from build123d import *

# Parameters (mm, degrees)
SKETCH1_W           = 152.25
SKETCH1_H           = 51
SKETCH1_R           = 1.75
SKETCH1_R_2         = 2
BOSS_EXTRUDE1_DEPTH = 1.5


with BuildPart() as part:
    # Sketch1 → Boss-Extrude1 (new body)
    with BuildSketch(Plane(origin=(0, 0, 0), x_dir=(1, 0, 0), z_dir=(0, 1, 0))):
        Rectangle(SKETCH1_W, SKETCH1_H)
        with Locations(Location((-63.125, 12.5, 0), (0, 0, 270))):
            Circle(SKETCH1_R, mode=Mode.SUBTRACT)
        with Locations(Location((-63.125, -13, 0), (0, 0, 270))):
            Circle(SKETCH1_R, mode=Mode.SUBTRACT)
        with Locations(Location((-28.125, 12.5, 0), (0, 0, 270))):
            Circle(SKETCH1_R, mode=Mode.SUBTRACT)
        with Locations(Location((-28.125, -13, 0), (0, 0, 270))):
            Circle(SKETCH1_R, mode=Mode.SUBTRACT)
        with Locations(Location((2.125, 12.5, 0), (0, 0, 270))):
            Circle(SKETCH1_R, mode=Mode.SUBTRACT)
        with Locations(Location((37.125, 12.5, 0), (0, 0, 270))):
            Circle(SKETCH1_R, mode=Mode.SUBTRACT)
        with Locations(Location((37.125, -13, 0), (0, 0, 270))):
            Circle(SKETCH1_R, mode=Mode.SUBTRACT)
        with Locations(Location((2.125, -13, 0), (0, 0, 270))):
            Circle(SKETCH1_R, mode=Mode.SUBTRACT)
        with Locations(Location((-71.125, 20.5, 0), (0, 0, 270))):
            Circle(SKETCH1_R_2, mode=Mode.SUBTRACT)
        with Locations(Location((71.125, 20.5, 0), (0, 0, 270))):
            Circle(SKETCH1_R_2, mode=Mode.SUBTRACT)
        with Locations(Location((71.125, -20.5, 0), (0, 0, 270))):
            Circle(SKETCH1_R_2, mode=Mode.SUBTRACT)
        with Locations(Location((-71.125, -20.5, 0), (0, 0, 270))):
            Circle(SKETCH1_R_2, mode=Mode.SUBTRACT)
    extrude(amount=-BOSS_EXTRUDE1_DEPTH)


solid = part.part
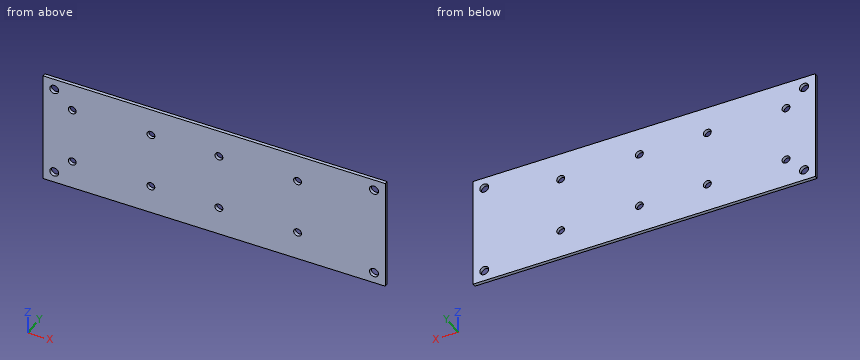
Here's how the part is built. I have some questions about the finished solid (model axes, mm). Round coordinates to 2 decimals unless told otherwise and drop trailing zeros. Loops run counter-clockwise (first coordinate to the right, second up) from the corner with the lowest first, then second, coordinate; pieces in that order, holes last. Notation, with made-up numbers: M 43,37.5 L 74,37.5 A13 cw 74,62.5 Z; hole C -8.75,84 d2. An arc over 180 degrees is marked long. Write each question's results on one line, items separated by ' | '. Start each with the question number.
(1) I want a section at B-B (z = 20.5). Please give me the cut outline in (x, y) (3 decimals), then the cut area to 3 significant figures.
(2) I want a section at C-C (y = -0.6). State how many separate pieces and enclosed holes the cut face has, then the cut area to 3 significant figures.
(3) Will these pins go through, and if not, where does the flat tip stop? P1, Ø2, axis at x = -28.125, z = 13, coming from the -Y side; P2, Ø6.5, axis at x = 71.125, z = 20.5, coming from the +Y side.
(4) If I drill on probe 1 along X at (y, z) = (-0.4, 13) (3 decimals); probe 2 along X at (y, z) = (-0.4, -21) (1 decimal); probe 3 along X at (y, z) = (-0.8, 14.5) (3 decimals), over which ranges is the centre line in solid material (lowest first)? Write a range as from..to.
(5) I want a section at A-A (z = -12.5). Please give me the cut outline in (x, y) (3 decimals), then the cut area to 3 significant figures.
Solved:
1) outline: M -76.125,-1.5 L -73.125,-1.5 L -73.125,0 L -76.125,0 Z; M -69.125,-1.5 L 69.125,-1.5 L 69.125,0 L -69.125,0 Z; M 73.125,-1.5 L 76.125,-1.5 L 76.125,0 L 73.125,0 Z | area: 216 mm²
2) separate pieces: 1 | enclosed holes: 12 | area: 7,640 mm²
3) P1: passes through | P2: stops at y = 0
4) probe 1: x = -76.125..-64.875, -61.375..-29.875, -26.375..0.375, 3.875..35.375, 38.875..76.125 | probe 2: x = -76.1..-73.1, -69.2..69.2, 73.1..76.1 | probe 3: x = -76.125..-64.026, -62.224..-29.026, -27.224..1.224, 3.026..36.224, 38.026..76.125
5) outline: M -76.125,-1.5 L -64.875,-1.5 L -64.875,0 L -76.125,0 Z; M -61.375,-1.5 L -29.875,-1.5 L -29.875,0 L -61.375,0 Z; M -26.375,-1.5 L 0.375,-1.5 L 0.375,0 L -26.375,0 Z; M 3.875,-1.5 L 35.375,-1.5 L 35.375,0 L 3.875,0 Z; M 38.875,-1.5 L 76.125,-1.5 L 76.125,0 L 38.875,0 Z | area: 207 mm²
